Could you check a few things on this model? Use its own coordinates, in mm. Give positions to 0.01 mm unless a question says otherwise; leave off trailing zeros. Loops run counter-clockwise (first coordinate to the right, second up) from the corner with the lowest first, then second, coordinate; pieces in that order, holes last. Notation, with made-up numbers: M -14,58 L -7,58 A26 cw -7,81 Z; hole C 31,81 d5. An arc over 180 degrees is marked long. Return JSON: item names as keys, results as strings. Group by question number.
1. If we section it at C-C (z = -7): Write out the boundary of the cut face in (x, y), plus the area to 3 significant figures.
2. If we mould it in two halves opening along Z, with no side actions, what happens to faces 1 (the cylindrical face through (17.448, 0.178, 14.646)), 2 (the cylindrical face through (-23.589, 0.178, 20.315)), 3 (the flat face through (0, 12.7, -15))? For each: +Z half, -Z half, draft (parallel to the pull), parting line (faces both ways), or undercut.
3. If we section it at B-B (y = -7.25): State how many separate pieces and enclosed holes the cut face has, plus the area to 3 significant figures.
4. Please list where these lines run through material, in increasing order: line 1 (Z direction, x = 19, y = 4.25) (3 decimals); line 2 (Z direction, x = 0, y = 4) (3 decimals); line 3 (X direction, y = -7.25, z = 2).
5. If we section it at A-A (x = 0): Write out the boundary of the cut face in (y, z) (3 decimals), plus the area to 3 significant figures.
```python
from build123d import *

# Parameters (mm, degrees)
F0_W     = 50.8
F0_H     = 44.45
F0_R     = 2.0193
F0_R_2   = 14.2875
F1_DEPTH = 12.7
F2_R     = 6.35


with BuildPart() as f1:
    # F0 (on Front) → F1 (new body, symmetric)
    with BuildSketch(Plane.XZ):
        Rectangle(F0_W, F0_H)
        with Locations((-19.05, -15.875)):
            Circle(F0_R, mode=Mode.SUBTRACT)
        with Locations((19.05, -15.875)):
            Circle(F0_R, mode=Mode.SUBTRACT)
        with Locations((0, 2.38125)):
            Circle(F0_R_2, mode=Mode.SUBTRACT)
        with Locations((-19.05, 15.875)):
            Circle(F0_R, mode=Mode.SUBTRACT)
        with Locations((19.05, 15.875)):
            Circle(F0_R, mode=Mode.SUBTRACT)
    extrude(amount=F1_DEPTH, both=True)

    # F2
    f2_edges = [f1.edges().sort_by_distance(p)[0] for p in [
        (25.4, 0, -22.225),
        (25.4, 0, 22.225),
        (-25.4, 0, 22.225),
        (-25.4, 0, -22.225),
    ]]
    fillet(f2_edges, radius=F2_R)


solid = f1.part
```
Answer:
{
 "1": {"outline": "M -25.4,-12.7 L -10.78,-12.7 L -10.78,12.7 L -25.4,12.7 Z; M 10.78,-12.7 L 25.4,-12.7 L 25.4,12.7 L 10.78,12.7 Z", "area": "743 mm²"},
 "2": {"face 1": "undercut", "face 2": "+Z half", "face 3": "draft"},
 "3": {"separate pieces": "1", "enclosed holes": "5", "area": "1,530 mm²"},
 "4": {"line 1": "z = -22.225 to -17.894, -13.856 to 13.856, 17.894 to 22.225", "line 2": "z = -22.225 to -11.906, 16.669 to 22.225", "line 3": "x = -25.4 to -14.28, 14.28 to 25.4"},
 "5": {"outline": "M -12.7,-22.225 L 12.7,-22.225 L 12.7,-11.906 L -12.7,-11.906 Z; M -12.7,16.669 L 12.7,16.669 L 12.7,22.225 L -12.7,22.225 Z", "area": "403 mm²"}
}
